Can you work these out from the model? Positions are in its coordinate system, mm. A direction names the side the tool comes from. Coordinates: 2 decimals unless noted, no trailing zeros. Order: outer loops, then holes, each group sorted by start corner. A loop starts at its lowest first (then second) coordinate and runs counter-clockwise, first axis right, second up. Notation, with made-up numbers: (14, 27) - (38, 27) arc R12 ccw to (38, 41) - close; hole circle Ø10 at (58, 28.5). An arc over 180 degrees is marked (long way). Use a Markdown table: item, result. Add a question column.
(1) I want a section at A-A (x = 0). List the corners of the cut face in (y, z) for me, and give its area (3 significant figures).
(2) I want a section at C-C (z = 108). List the corners of the cut face in (x, y) for me.
(3) For pin 1 Ø4 at (x, y) = (1.5, -12) entering from -Z; pin 2 Ø20 at (x, y) = (-9, 9.5) entering from +Z; pin 3 Ø2 at (y, z) = (-14, 9) entering from -X; pin 4 Ø6 at (y, z) = (-11, 28.5) entering from -X, each with a flat end and sliding along its axis, tell me the tip position at first contact or that it passes through.
(4) I want a section at D-D (y = 16). List the corners of the cut face in (x, z) for me, and give its area (3 significant figures).
(5) If I drill on L1, parallel to Z at x = -11, y = -7; L2, parallel to Y at x = -0.5, z = 21; L3, parallel to X at y = -10, z = 69, over which ranges is the centre line in solid material (lowest first)? Write a range as [from, to].
(6) On a 3-axis mill with a long thin cutter (end or side, diameter ignored), from which of +Z, -Z, +X, -X, +Y, -Y can I reach the whole of each face in a straight line? I mean faces 1 (the flat face through (4, -4, 100)), 2 (the flat face through (4, -4, 0)), 3 (the flat face through (0, 0, -20)). Say none if no direction works.
```python
from build123d import *

# Parameters (mm, degrees)
SKETCH1_R           = 20
BOSS_EXTRUDE1_DEPTH = 100
SKETCH2_R           = 5
BOSS_EXTRUDE2_DEPTH = 30
LPATTERN1_COUNT     = 2
LPATTERN1_PITCH     = 130
SKETCH3_R           = 7.5
CUT_EXTRUDE1_DEPTH  = 10


with BuildPart() as part:
    # Sketch1 → Boss-Extrude1 (new body)
    with BuildSketch(Plane.XY):
        Circle(SKETCH1_R)
    extrude(amount=BOSS_EXTRUDE1_DEPTH)

    # Sketch2 → Boss-Extrude2 (add)
    with BuildSketch(Plane.XY.offset(100)):
        with Locations(Location((0, 0, 0), (0, 0, 180))):
            Circle(SKETCH2_R)
    boss_extrude2 = extrude(amount=BOSS_EXTRUDE2_DEPTH)

    # LPattern1: Boss-Extrude2 ×2
    with Locations(*[(0, 0, -i * LPATTERN1_PITCH) for i in range(1, LPATTERN1_COUNT)]):
        add(boss_extrude2)

    # Sketch3 → Cut-Extrude1 (cut)
    with BuildSketch(Plane(origin=(0, 0, -30), x_dir=(-1, 0, 0), z_dir=(0, 0, -1))):
        Circle(SKETCH3_R)
    extrude(amount=-CUT_EXTRUDE1_DEPTH, mode=Mode.SUBTRACT)


solid = part.part
```
Answers follow:
| question | item | result |
|---|---|---|
| 1 | outline | (-20, 0) - (-5, 0) - (-5, -20) - (5, -20) - (5, 0) - (20, 0) - (20, 100) - (5, 100) - (5, 130) - (-5, 130) - (-5, 100) - (-20, 100) - close |
| 1 | area | 4,500 mm² |
| 2 | outline | circle Ø10 at (0, 0) |
| 3 | pin 1 | stops at z = 0 |
| 3 | pin 2 | stops at z = 130 |
| 3 | pin 3 | stops at x = -15.2 |
| 3 | pin 4 | stops at x = -18.33 |
| 4 | outline | (-12, 0) - (12, 0) - (12, 100) - (-12, 100) - close |
| 4 | area | 2,400 mm² |
| 5 | L1 | z = [0, 100] |
| 5 | L2 | y = [-19.99, 19.99] |
| 5 | L3 | x = [-17.32, 17.32] |
| 6 | face 1 | +Z |
| 6 | face 2 | -Z |
| 6 | face 3 | -Z, +X, -X, +Y, -Y |
